Verification items for the finished model (mm, model axes). Round coordinates to 2 decimals unless told otherwise and drop trailing zeros. Write each loop counter-clockwise with the first axis right and the second up, starting at its lowest first coordinate (ties: lowest second). Pieces come first, ordered by that corner, then holes. Notation, with made-up numbers: M 88.5,85.5 L 114.5,85.5 A22 cw 114.5,106.5 Z; hole C 67,-15.75 d1. An arc over 180 degrees is marked long. Answer in a Markdown table with one row per item. Add a question column.
1. Sectioned sample at A-A on x = 109. Record the cut outline in (y, z).
2. Go/stop test with flat-tipped pins: pin 1 Ø6.5 at (x, z) = (-59.5, 4) entering from -Y; pin 2 Ø2.5 at (x, y) = (-151, 20.5) entering from -Z; pin 3 Ø9.5 at (x, y) = (58.5, 45.5) entering from -Z. Record where each tip stops, or that it passes through.
3. Sectioned sample at C-C on z = 3.5. Record the cut outline in (x, y).
4. Material ranges on probe 1 along Y at (x, z) = (-113, 3.25); probe 2 along Y at (x, z) = (150, 3.5); probe 3 along Z at (x, y) = (-49, 43), recorded low to high.
5. Sectioned sample at B-B on y = 42.5. Record the cut outline in (x, z), plus the area to 4 significant figures.
```python
from build123d import *

# Parameters (mm, degrees)
SK_BODY_W               = 324
SK_BODY_H               = 90
EX_BODY_DEPTH           = 15
SK_SWITCHPOCKETS_W      = 20
SK_SWITCHPOCKETS_H      = 12
CUT_SWITCHPOCKETS_DEPTH = 8
SK_GUIDEPINS_R          = 2.5
CUT_GUIDEPINS_DEPTH     = 10
SK_CLIFFWINDOWS_W       = 58.5
SK_CLIFFWINDOWS_H       = 31.552578851
CUT_CLIFFWINDOWS_DEPTH  = 15


with BuildPart() as part:
    # SK_Body → EX_Body (new body)
    with BuildSketch(Plane.XY):
        with Locations((0, 45)):
            Rectangle(SK_BODY_W, SK_BODY_H)
    extrude(amount=EX_BODY_DEPTH)

    # SK_SwitchPockets → CUT_SwitchPockets (cut)
    with BuildSketch(Plane.XY):
        with Locations((55, 45)):
            Rectangle(SK_SWITCHPOCKETS_W, SK_SWITCHPOCKETS_H)
        with Locations((-55, 45)):
            Rectangle(SK_SWITCHPOCKETS_W, SK_SWITCHPOCKETS_H)
    extrude(amount=CUT_SWITCHPOCKETS_DEPTH, mode=Mode.SUBTRACT)

    # SK_GuidePins → CUT_GuidePins (cut)
    with BuildSketch(Plane.XY):
        with Locations((150, 20)):
            Circle(SK_GUIDEPINS_R)
        with Locations((-150, 20)):
            Circle(SK_GUIDEPINS_R)
    extrude(amount=CUT_GUIDEPINS_DEPTH, mode=Mode.SUBTRACT)

    # SK_CliffWindows → CUT_CliffWindows (cut)
    with BuildSketch(Plane.XY):
        with Locations((100.25, 35.723710575)):
            Rectangle(SK_CLIFFWINDOWS_W, SK_CLIFFWINDOWS_H)
        with Locations((-100.25, 35.723710575)):
            Rectangle(SK_CLIFFWINDOWS_W, SK_CLIFFWINDOWS_H)
    extrude(amount=CUT_CLIFFWINDOWS_DEPTH, mode=Mode.SUBTRACT)


solid = part.part
```
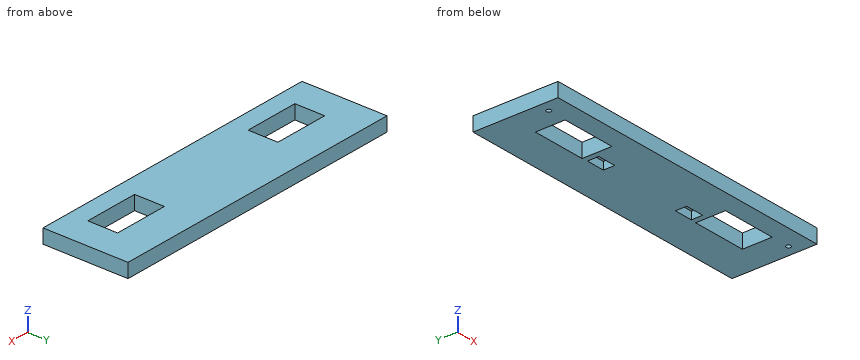
Geometry check:
| question | item | result |
|---|---|---|
| 1 | outline | M 0,0 L 19.95,0 L 19.95,15 L 0,15 Z; M 51.5,0 L 90,0 L 90,15 L 51.5,15 Z |
| 2 | pin 1 | stops at y = 0 |
| 2 | pin 2 | stops at z = 10 |
| 2 | pin 3 | stops at z = 8 |
| 3 | outline | M -162,0 L 162,0 L 162,90 L -162,90 Z; hole C -150,20 d5; hole M -129.5,19.95 L -71,19.95 L -71,51.5 L -129.5,51.5 Z; hole M -65,39 L -45,39 L -45,51 L -65,51 Z; hole M 45,39 L 65,39 L 65,51 L 45,51 Z; hole M 71,19.95 L 129.5,19.95 L 129.5,51.5 L 71,51.5 Z; hole C 150,20 d5 |
| 4 | probe 1 | y = 0 to 19.95, 51.5 to 90 |
| 4 | probe 2 | y = 0 to 17.5, 22.5 to 90 |
| 4 | probe 3 | z = 8 to 15 |
| 5 | outline | M -162,0 L -129.5,0 L -129.5,15 L -162,15 Z; M -71,0 L -65,0 L -65,8 L -45,8 L -45,0 L 45,0 L 45,8 L 65,8 L 65,0 L 71,0 L 71,15 L -71,15 Z; M 129.5,0 L 162,0 L 162,15 L 129.5,15 Z |
| 5 | area | 2,785 mm2 |
